Autodesk Inventor part; units mm, degrees
ref_plane "side_1_XY" through (0, -18.25, 0) normal (0, -1, 0) x (1, 0, 0)
ref_plane "side_1_YZ" through (0, -18.25, 0) normal (1, 0, 0) x (0, 0, 1)
ref_plane "side_1_ZX" through (0, -18.25, 0) normal (0, 0, 1) x (0, -1, 0)
sketch "Sketch_1" plane through (0, 0, 0) normal (1, 0, 0) x (0, 1, 0)
  line L0 (0, -50) -> (0, 50)
  circle A0 centre (15.75, 0) radius 3
revolve "Revolution1" add sketch "Sketch_1" angle 360 about axis through (0, 0, -50) along (0, 0, -1)
sketch "Sketch_3" plane through (0, 0, 0) normal (0, 0, 1) x (1, 0, 0)
  line L0 (-20, -23.25) -> (20, -23.25)
  line L1 (20, -23.25) -> (20, -18.25)
  line L2 (20, -18.25) -> (-20, -18.25)
  line L3 (-20, -18.25) -> (-20, -23.25)
sketch "Sketch_2" plane through (0, 0, 0) normal (0, 0, 1) x (1, 0, 0)
  line L0 (-10, -18.25) -> (10, -18.25)
  line L1 (10, -18.25) -> (10, -12.25)
  line L2 (10, -12.25) -> (-10, -12.25)
  line L3 (-10, -12.25) -> (-10, -18.25)
extrude "Extrusion1" add sketch "Sketch_2" along normal mid plane 11
extrude "Extrusion2" cut sketch "Sketch_3" along normal mid plane 11
sketch "Sketch_4" plane through (0, 0, 0) normal (1, 0, 0) x (0, 1, 0)
  line L0 (-50, 0) -> (50, 0)
  line L1 (-7.25, 0) -> (-7.25, -5)
  line L2 (-7.25, -5) -> (-12.25, -5)
  line L3 (-12.25, -5) -> (-14.6, -2.65)
  line L4 (-14.6, -2.65) -> (-18.25, -2.65)
  line L5 (-18.25, -2.65) -> (-18.25, 0)
  line L6 (-18.25, 0) -> (-7.25, 0)
revolve "Revolution2" cut sketch "Sketch_4" angle 360 about axis through (0, -50, 0) along (0, -1, 0)
sketch "Sketch_5" plane through (0, 0, 0) normal (1, 0, 0) x (0, 1, 0)
  line L0 (-26.25, 0) -> (-12.25, 0)
  line L1 (-12.25, 0) -> (-12.25, -4.95)
  line L2 (-12.25, -4.95) -> (-14.96, -2.5)
  line L3 (-14.96, -2.5) -> (-25.7595, -2.5)
  line L4 (-25.7595, -2.5) -> (-26.25, -2.0095)
  line L5 (-26.25, -2.0095) -> (-26.25, 0)
  line L6 (-26.25, 0) -> (-12.25, 0)
revolve "Revolution3" add sketch "Sketch_5" angle 360 about axis through (0, -26.25, 0) along (0, -1, 0)
thread "Thread1"
sketch "Sketch_6" plane through (0, -12.25, 0) normal (0, 1, 0) x (0, 0, -1)
  line L0 (-1.5, 0.866) -> (-1.5, -0.866)
  line L1 (-1.5, -0.866) -> (0, -1.7321)
  line L2 (0, -1.7321) -> (1.5, -0.866)
  line L3 (1.5, -0.866) -> (1.5, 0.866)
  line L4 (1.5, 0.866) -> (0, 1.7321)
  line L5 (0, 1.7321) -> (-1.5, 0.866)
extrude "Extrusion3" cut sketch "Sketch_6" against normal blind 2
ref_plane "side_1_XY" through (0, -18.25, 0) normal (0, -1, 0) x (1, 0, 0)
ref_plane "side_1_YZ" through (0, -18.25, 0) normal (1, 0, 0) x (0, 0, 1)
ref_plane "side_1_ZX" through (0, -18.25, 0) normal (0, 0, 1) x (0, -1, 0)
properties part number "May Tec 1.71.30365_Installation ring_36.5"
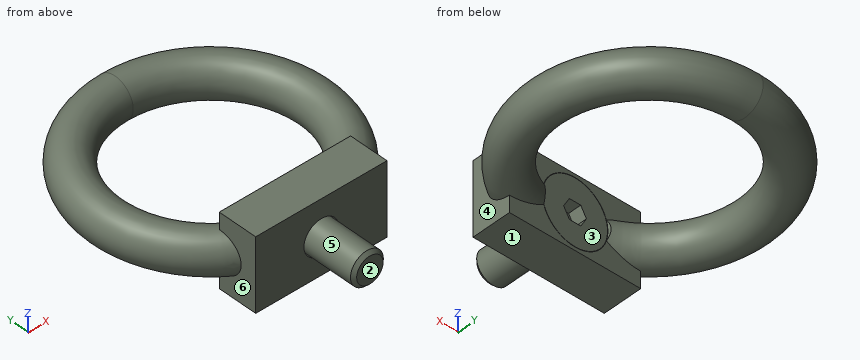
The listing builds one solid part. Answer for the finished solid, in the listing's coordinates (mm). Face numbers are marked on the shaded views. A direction names the side the tool comes from. Give positions to 0.01 mm unless a question says otherwise; leave off trailing zeros.
Item 1: Find the intervals of material crossed by line 1 along X through (y, z) = (4.5, 1.5); line 2 along X through (y, z) = (0, -1.75); line 3 along Y through (x, z) = (-9.5, 4.75), in increasing order.
Derived:
line 1: x = -17.79 to -12.36, 12.36 to 17.79
line 2: x = -18.19 to -13.31, 13.31 to 18.19
line 3: y = -18.25 to -12.25
Item 2: A tool of negligible diameter and unlimited length cuts with its end or side. For the marked faces 4, 5 and 6, from which of +Z, -Z, +X, -X, +Y, -Y can it reach the whole face along a straight path? Write none if from no direction.
Derived:
face 4: +X, -Y
face 5: -Y
face 6: -X, -Y
Item 3: Each of these flat-tipped pins is pushed along its axis until it touches: pin 1 Ø2 at (x, z) = (0, -4.5) entering from +Y; pin 2 Ø5 at (x, y) = (-14, -15.5) entering from -Z; pin 3 Ø1.8 at (y, z) = (-14, 1.5) entering from +X; pin 4 Ø1 at (y, z) = (9, -4.5) entering from +X. Where does it stop, or does it pass through?
Derived:
pin 1: stops at y = -12.25
pin 2: stops at z = -1.43
pin 3: stops at x = 13.03
pin 4: passes through
Item 4: Determine the mould class of the marked faces 1, 2 and 3 for opening direction Y: +Y half, -Y half, draft (parallel to the pull), parting line (faces both ways), or undercut.
Derived:
face 1: draft
face 2: -Y half
face 3: undercut
